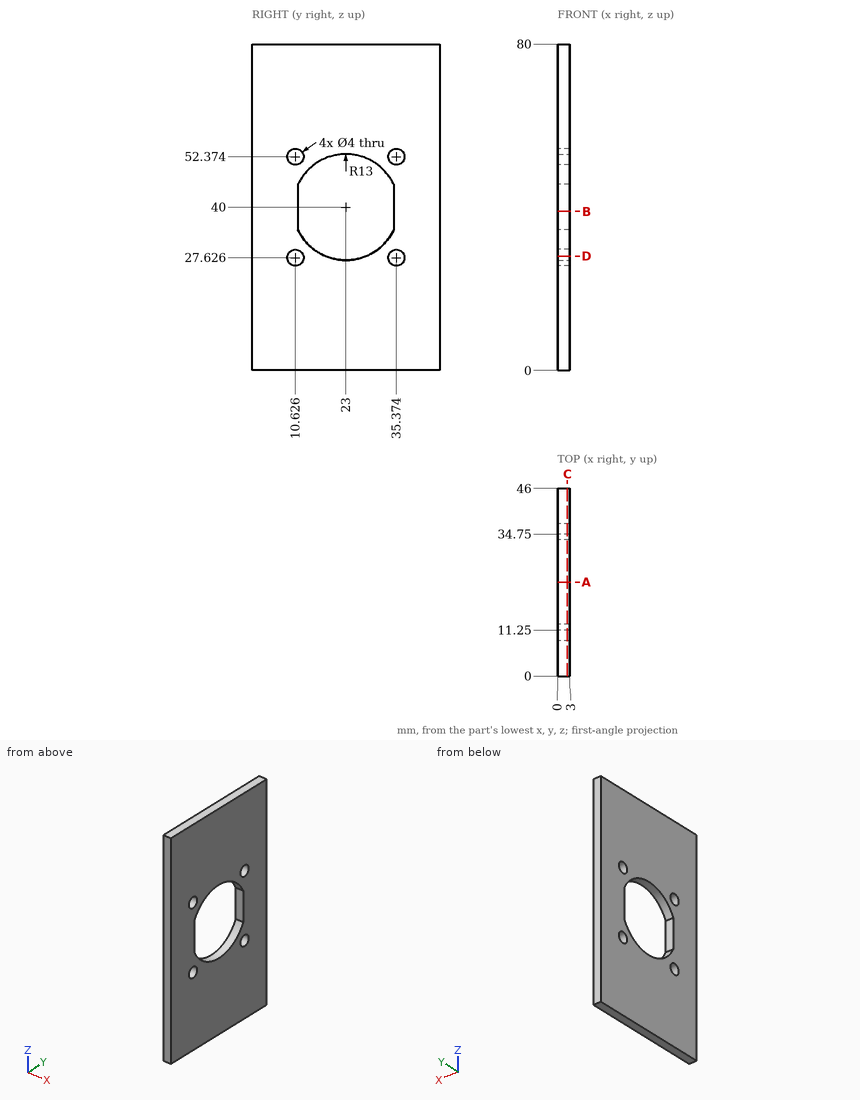
Verification items for this drawing (mm, ordinates from the low corner). Give positions to 0.01 mm unless a question says otherwise; leave off trailing zeros. Write each loop counter-clockwise with the first axis right and the second up, starting at its lowest first coordinate (ties: lowest second). Pieces come first, ordered by that corner, then holes. Notation, with made-up numbers: (-29, -16.75) - (15, -16.75) arc R22 cw to (15, 12.25) - close; hole circle Ø11 at (87.5, 16.5). An arc over 180 degrees is marked (long way). Answer as a JSON object with one key per item and string values. Group by question number.
1) Sectioned sample at B-B (z = 39). Record the cut outline in (x, y), then the cut area to 3 significant figures.
2) Thickness scan on probe 1 along Z at (x, y) = (0.9, 22.5); probe 2 along Y at (x, z) = (1.7, 28) (1 decimal); probe 3 along Y at (x, z) = (0.95, 28.5) (1 decimal). Record the ranges inside material, lowest first. Write a range as from..to.
3) Sectioned sample at D-D (z = 28). Record the cut outline in (x, y).
4) Depth check by flat-ended pin: P1, Ø2.5, axis at y = 10.63, z = 52.37, coming from the +X side. Enter the tip coordinate at first touch or a pass-through.
5) Sectioned sample at C-C (x = 2.35). Give the number of separate pieces and of enclosed holes in the cut face, then the cut area to 3 significant figures.
6) Sectioned sample at A-A (y = 23). Record the cut outline in (x, z), then the cut area to 3 significant figures.
Geometry results:
{
 "1": {"outline": "(0, 0) - (3, 0) - (3, 11.25) - (0, 11.25) - close; (0, 34.75) - (3, 34.75) - (3, 46) - (0, 46) - close", "area": "67.5 mm^2"},
 "2": {"probe 1": "z = 0..27.01, 52.99..80", "probe 2": "y = 0..8.7, 12.6..18, 28..33.4, 37.3..46", "probe 3": "y = 0..8.8, 12.4..16.9, 29.1..33.6, 37.2..46"},
 "3": {"outline": "(0, 0) - (3, 0) - (3, 8.66) - (0, 8.66) - close; (0, 12.59) - (3, 12.59) - (3, 18) - (0, 18) - close; (0, 28) - (3, 28) - (3, 33.41) - (0, 33.41) - close; (0, 37.34) - (3, 37.34) - (3, 46) - (0, 46) - close"},
 "4": {"P1": "passes through"},
 "5": {"separate pieces": "1", "enclosed holes": "5", "area": "3,120 mm^2"},
 "6": {"outline": "(0, 0) - (3, 0) - (3, 27) - (0, 27) - close; (0, 53) - (3, 53) - (3, 80) - (0, 80) - close", "area": "162 mm^2"}
}
